Source: CAD feature listing. Evaluate the final solid. Frame: model axes, mm. A direction names the side the tool comes from. Round coordinates to 2 decimals unless told otherwise and drop trailing zeros. Write each loop counter-clockwise with the first axis right and the second up, starting at its lowest first coordinate (ties: lowest second). Pieces come first, ordered by that corner, then holes.
from build123d import *

# Parameters (mm, degrees)
F1_DEPTH = 25
F2_DEPTH = 10
F3_DEPTH = 3.125
F5_R     = 2.5


with BuildPart() as f1:
    # F0 (on Front) → F1 (new body, symmetric)
    with BuildSketch(Plane.XZ):
        Polygon((8.75, 3.75), (-16.25, 3.75), (-16.25, -3.75), (16.25, -3.75), (16.25, 3.75), align=None)
    extrude(amount=F1_DEPTH, both=True)

    # F0 (on Front) → F2 (join, symmetric)
    with BuildSketch(Plane.XZ):
        with BuildLine():
            Line((8.75, 10.63), (8.75, 3.75))
            Line((8.75, 3.75), (16.25, 3.75))
            Line((16.25, 3.75), (16.25, 10.63))
            ThreePointArc((16.25, 10.63), (18.080583, 15.049417), (22.5, 16.88))
            Line((22.5, 16.88), (23.75, 16.88))
            Line((23.75, 16.88), (23.75, 24.38))
            Line((23.75, 24.38), (22.5, 24.38))
            ThreePointArc((22.5, 24.38), (12.777282, 20.352718), (8.75, 10.63))
        make_face()
        Polygon((33.742055, 24.38), (23.75, 24.38), (23.75, 16.88), (23.75, 15), (33.742055, 15), align=None)
    extrude(amount=F2_DEPTH, both=True)

    # F0 (on Front) → F3 (join, symmetric)
    with BuildSketch(Plane.XZ):
        with BuildLine():
            add(Edge.make_bspline(
                [(-16.25, 3.75), (-9.499033, 16.007805), (3.585062, 26.59969), (22.5, 24.38)],
                knots=[0, 0, 0, 0, 43.899424, 43.899424, 43.899424, 43.899424], degree=3))
            Line((-16.25, 3.75), (8.75, 3.75))
            Line((8.75, 3.75), (8.75, 10.63))
            ThreePointArc((8.75, 10.63), (12.777282, 20.352718), (22.5, 24.38))
        make_face()
    extrude(amount=F3_DEPTH, both=True)

    # F0 (on Front) → F4 (revolve)
    with BuildSketch(Plane.XZ):
        Polygon((33.742055, 26.25), (33.742055, 24.38), (33.742055, 15), (43.75, 15), (43.75, 26.25), align=None)
    revolve(axis=Axis((33.742055, 0, 20.625), (0, 0, -1)))

    # F5
    f5_edges = [f1.edges().sort_by_distance(p)[0] for p in [
        (16.25, 25, 0),
        (-16.25, 25, 0),
        (-16.25, -25, 0),
        (16.25, -25, 0),
    ]]
    fillet(f5_edges, radius=F5_R)


solid = f1.part
1) Material intervals for line 1 (Z direction, x = 6, y = 19); line 2 (Y direction, x = -7, z = 9) (3 decimals); line 3 (X direction, y = 5.5, z = 15.5), sorted ascending.
Taken from the geometry:
line 1: z = -3.75 to 3.75
line 2: y = -3.125 to 3.125
line 3: x = 9.64 to 18.58, 23.75 to 42.1
2) Pull-direction query (X, two-part tool) for faces 1 (the face through (34, 0, 26.25)), 2 (the face through (18.03, -0.14, 15)), 3 (the face through (8.75, 7, 7)), 4 (the face through (23.5, 1.4, 24.38)); classes: released by +X, released by -X, zero draft, split by the parting line, or undercut.
Taken from the geometry:
face 1: zero draft
face 2: undercut
face 3: released by -X
face 4: undercut
3) Contact query for flat-ended pins moving along their axis: P1, Ø10, axis at x = 32, z = 11, coming from the +Y side; P2, Ø6, axis at y = -14.5, z = 16.5, coming from the +X side; P3, Ø10, axis at x = 37, y = 14.5, coming from the -Z side; P4, Ø0.6, axis at y = -3.5, z = 16, coming from the -X side. Output: stop coordinate, or through.
Taken from the geometry:
P1: stops at y = 10.01
P2: passes through
P3: stops at z = 15
P4: stops at x = 9.72
4) Section query B-B on y = 16. Return the cut outline in (x, z), then the cut area to 3 significant figures.
Taken from the geometry:
outline: (-16.25, -3.75) - (16.25, -3.75) - (16.25, 3.75) - (-16.25, 3.75) - close
area: 244 mm2
5) Section query A-A on z = 2.5. Return the cut outline in (x, y), then the cut area to 3 significant figures.
Taken from the geometry:
outline: (-16.25, -22.5) arc R2.5 ccw to (-13.75, -25) - (13.75, -25) arc R2.5 ccw to (16.25, -22.5) - (16.25, 22.5) arc R2.5 ccw to (13.75, 25) - (-13.75, 25) arc R2.5 ccw to (-16.25, 22.5) - close
area: 1,620 mm2
6) Reachability of faces 5 (the face through (16.25, 0, 2)), 6 (the face through (43, 3.8, 22)), 7 (the face through (18, 10, 17)), 8 (the face through (12.885, 6.514, 20.459)) from +Z, -Z, +X, -X, +Y, -Y: full face, straight path, thin tool, end or side. Return the list, or none.
Taken from the geometry:
face 5: -Z, +X, +Y, -Y
face 6: +Z
face 7: +Z, +X, -X, +Y
face 8: +Z, -X, +Y
7) Section query C-C on x = 38.5. Return the cut outline in (y, z), then the cut area to 3 significant figures.
Taken from the geometry:
outline: (-8.8, 15) - (8.8, 15) - (8.8, 26.25) - (-8.8, 26.25) - close
area: 198 mm2
